Read the model definition and answer for the solid it produces. Units are mm, in the model's axes. A direction names the side the tool comes from. Round coordinates to 2 decimals unless told otherwise and drop trailing zeros. Order: outer loops, then holes, each group sorted by start corner. A loop starts at its lowest first (then second) coordinate and runs counter-clockwise, first axis right, second up. Notation, with made-up numbers: (-25.75, 80) -> (-5.75, 80) arc R20 ccw to (-5.75, 105) -> close; hole circle Ø4 at (24.25, 17.25). An arc over 180 degrees is marked (long way). Use a Markdown table: item, result. Add a question column.
1. Section B-B, the plane y = -12 is taken. Give the vertices of the cut face in (x, z), then the cut area to 3 significant figures.
2. Section C-C, the plane x = 1 is taken. Give the vertices of the cut face in (y, z).
3. For faces 4 (the face through (-14, 19, 10)), 5 (the face through (20, 19, 10)), 6 (the face through (-23, 10, 10)), 7 (the face through (20, 15, 10)), determine the directions among +Z, -Z, +X, -X, +Y, -Y from which every point of the face is accessible in a straight line to the end or side of a thin tool.
4. Consider L1, parallel to X at y = 26.45, z = 10; L2, parallel to Y at x = 9, z = 19.25; L3, parallel to X at y = -11, z = 17.5. Determine where each line is inside the solid, lowest interval first. Write a range as [from, to].
5. Given pin 1 (2 mm diameter, centred on x = 21.5, y = -12, fed in from +Z); pin 2 (11 mm diameter, centred on x = -2.5, y = -4, fed in from -Z); pin 3 (4.5 mm diameter, centred on y = -13, z = 11, fed in from +X), each flat-ended and moving along its own axis, determine where each tip first touches the part or whether it passes through.
6. Section D-D, the plane y = 24.5 is taken. Give the vertices of the cut face in (x, z).
7. Section A-A, the plane x = -25 is taken. Give the vertices of the cut face in (y, z).
8. The mould has two halves that part along X. Classify faces 1 (the face through (-4, 19, 19)), 2 (the face through (11.352, 23.472, 14.292)), 3 (the face through (-23, 12, 16)): +X half, -X half, draft (parallel to the pull), parting line (faces both ways), or undercut.
```python
from build123d import *

# Parameters (mm, degrees)
SKETCH1_W           = 40
SKETCH1_H           = 36
BOSS_EXTRUDE1_DEPTH = 20
BOSS_EXTRUDE3_DEPTH = 2
SKETCH4_R           = 7
BOSS_EXTRUDE4_DEPTH = 1
SKETCH5_R           = 6
BOSS_EXTRUDE5_DEPTH = 0.5
SKETCH8_R           = 4.5
BOSS_EXTRUDE6_DEPTH = 4
SKETCH9_R           = 10.5
BOSS_EXTRUDE7_DEPTH = 2
SKETCH13_W          = 7
SKETCH13_H          = 3
BOSS_EXTRUDE8_DEPTH = 20
CUT_EXTRUDE1_DEPTH  = 3
SKETCH17_W          = 6
SKETCH17_H          = 4
BOSS_EXTRUDE9_DEPTH = 2
SKETCH19_R          = 1.05
CUT_EXTRUDE2_DEPTH  = 2


with BuildPart() as part:
    # Sketch1 → Boss-Extrude1 (new body)
    with BuildSketch(Plane.XY):
        Rectangle(SKETCH1_W, SKETCH1_H)
    extrude(amount=BOSS_EXTRUDE1_DEPTH)

    # Sketch2 → Boss-Extrude3 (add)
    with BuildSketch(Plane(origin=(0, 18, 0), x_dir=(1, 0, 0), z_dir=(0, 1, 0))):
        with BuildLine():
            Line((-14, -1), (5.641101056, -1))
            ThreePointArc((5.641101056, -1), (20, -10), (5.641101056, -19))
            Line((5.641101056, -19), (-14, -19))
            Line((-14, -19), (-14, -1))
        make_face()
    extrude(amount=BOSS_EXTRUDE3_DEPTH)

    # Sketch4 → Boss-Extrude4 (add)
    with BuildSketch(Plane(origin=(0, 20, 0), x_dir=(1, 0, 0), z_dir=(0, 1, 0))):
        with Locations(Location((10, -10, 0), (0, 0, 270))):
            Circle(SKETCH4_R)
    extrude(amount=BOSS_EXTRUDE4_DEPTH)

    # Sketch5 → Boss-Extrude5 (add)
    with BuildSketch(Plane(origin=(0, 21, 0), x_dir=(1, 0, 0), z_dir=(0, 1, 0))):
        with Locations(Location((10, -10, 0), (0, 0, 270))):
            Circle(SKETCH5_R)
    extrude(amount=BOSS_EXTRUDE5_DEPTH)

    # Sketch8 → Boss-Extrude6 (add)
    with BuildSketch(Plane(origin=(0, 21.5, 0), x_dir=(1, 0, 0), z_dir=(0, 1, 0))):
        with Locations(Location((10, -10, 0), (0, 0, 270))):
            Circle(SKETCH8_R)
    extrude(amount=BOSS_EXTRUDE6_DEPTH)

    # Sketch9 → Boss-Extrude7 (add)
    with BuildSketch(Plane(origin=(0, 25.5, 0), x_dir=(1, 0, 0), z_dir=(0, 1, 0))):
        with Locations(Location((10, -10, 0), (0, 0, 270))):
            Circle(SKETCH9_R)
    extrude(amount=BOSS_EXTRUDE7_DEPTH)

    # Sketch13 → Boss-Extrude8 (add)
    with BuildSketch(Plane(origin=(0, 0, 0), x_dir=(-1, 0, 0), z_dir=(0, 0, -1))):
        with Locations((23.5, 11.5)):
            Rectangle(SKETCH13_W, SKETCH13_H)
        with Locations((-23.5, 11.5)):
            Rectangle(SKETCH13_W, SKETCH13_H)
    extrude(amount=-BOSS_EXTRUDE8_DEPTH)

    # Sketch14 → Cut-Extrude1 (cut)
    with BuildSketch(Plane(origin=(0, 13, 0), x_dir=(1, 0, 0), z_dir=(0, 1, 0))):
        with BuildLine():
            Line((-27, -17), (-27, -15))
            Line((-27, -15), (-26.732050808, -15))
            ThreePointArc((-26.732050808, -15), (-23, -16), (-26.732050808, -17))
            Line((-26.732050808, -17), (-27, -17))
        make_face()
        with BuildLine():
            Line((-27, -3), (-26.732050808, -3))
            ThreePointArc((-26.732050808, -3), (-23, -4), (-26.732050808, -5))
            Line((-26.732050808, -5), (-27, -5))
            Line((-27, -5), (-27, -3))
        make_face()
    cut_extrude1 = extrude(amount=-CUT_EXTRUDE1_DEPTH, mode=Mode.SUBTRACT)

    # Mirror2: Cut-Extrude1 across plane
    add(cut_extrude1.mirror(Plane(origin=(0, 0, 0), x_dir=(0, 0, 1), z_dir=(1, 0, 0))), mode=Mode.SUBTRACT)

    # Sketch17 → Boss-Extrude9 (add)
    with BuildSketch(Plane(origin=(20, 0, 0), x_dir=(0, 0, -1), z_dir=(1, 0, 0))):
        with Locations((-10, -13)):
            Rectangle(SKETCH17_W, SKETCH17_H)
    extrude(amount=BOSS_EXTRUDE9_DEPTH)

    # Sketch19 → Cut-Extrude2 (cut)
    with BuildSketch(Plane(origin=(0, 27.5, 0), x_dir=(1, 0, 0), z_dir=(0, 1, 0))):
        with Locations(Location((10, -3, 0), (0, 0, 270))):
            Circle(SKETCH19_R)
        with Locations(Location((3, -10, 0), (0, 0, 270))):
            Circle(SKETCH19_R)
        with Locations(Location((10, -17, 0), (0, 0, 90))):
            Circle(SKETCH19_R)
        with Locations(Location((17, -10, 0), (0, 0, 90))):
            Circle(SKETCH19_R)
    extrude(amount=-CUT_EXTRUDE2_DEPTH, mode=Mode.SUBTRACT)


solid = part.part
```
Verdict:
| question | item | result |
|---|---|---|
| 1 | outline | (-20, 0) -> (20, 0) -> (20, 7) -> (22, 7) -> (22, 13) -> (20, 13) -> (20, 20) -> (-20, 20) -> close |
| 1 | area | 812 mm2 |
| 2 | outline | (-18, 0) -> (18, 0) -> (18, 1) -> (20, 1) -> (20, 19) -> (18, 19) -> (18, 20) -> (-18, 20) -> close; (25.5, 4.59) -> (27.5, 4.59) -> (27.5, 15.41) -> (25.5, 15.41) -> close |
| 3 | face 4 | +Z, -Z, -X, +Y |
| 3 | face 5 | none |
| 3 | face 6 | +Z, -Z, -X, -Y |
| 3 | face 7 | +Z, -Z, +X |
| 4 | L1 | x = [-0.5, 1.95], [4.05, 15.95], [18.05, 20.5] |
| 4 | L2 | y = [-18, 20], [25.5, 27.5] |
| 4 | L3 | x = [-20, 20] |
| 5 | pin 1 | stops at z = 13 |
| 5 | pin 2 | stops at z = 0 |
| 5 | pin 3 | stops at x = 22 |
| 6 | outline | circle Ø9 at (10, 10) |
| 7 | outline | (10, 0) -> (13, 0) -> (13, 2) -> (10, 2) -> close; (10, 6) -> (13, 6) -> (13, 14) -> (10, 14) -> close; (10, 18) -> (13, 18) -> (13, 20) -> (10, 20) -> close |
| 8 | face 1 | draft |
| 8 | face 2 | parting line |
| 8 | face 3 | undercut |
